Autodesk Inventor part; units mm, degrees
ref_plane "YZ Plane" through (0, 0, 0) normal (1, 0, 0) x (0, 1, 0)
ref_plane "XZ Plane" through (0, 0, 0) normal (0, 1, 0) x (-1, 0, 0)
ref_plane "XY Plane" through (0, 0, 0) normal (0, 0, 1) x (1, 0, 0)
sketch "Sketch1" plane through (0, 0, 0) normal (0, 0, 1) x (1, 0, 0)
  line L0 (-5, 12.5) -> (5, 12.5)
  line L1 (5, 12.5) -> (5, 2.5)
  line L2 (5, 2.5) -> (-5, 2.5)
  line L3 (-5, 2.5) -> (-5, 12.5)
  line L4 (-6.5, 1) -> (-6.5, 14)
  line L5 (6.5, 1) -> (-6.5, 1)
  line L6 (6.5, 14) -> (6.5, 1)
  line L7 (-6.5, 14) -> (6.5, 14)
  line L8 (-5, 2.5) -> (5, 2.5)
  line L9 (5, 2.5) -> (5, 12.5)
  line L10 (5, 12.5) -> (-5, 12.5)
  line L11 (-5, 12.5) -> (-5, 2.5)
  line L12 (4.1303, 3.3697) -> (-4.1303, 3.3697)
  line L13 (-4.1303, 3.3697) -> (-4.1303, 11.6303)
  line L14 (-4.1303, 11.6303) -> (4.1303, 11.6303)
  line L15 (4.1303, 11.6303) -> (4.1303, 3.3697)
  line L16 (-4.1303, 3.3697) -> (4.1303, 11.6303) construction
  point P0 (0, 0)
  point P1 (0, 7.5)
extrude "Extrusion1" add sketch "Sketch1" along normal blind 30 contours L0 L1 L2 L3
sketch "Sketch2" plane through (0, 0, 30) normal (0, 0, 1) x (1, 0, 0)
  line L0 (-5, 2.5) -> (5, 2.5)
  line L1 (5, 2.5) -> (5, 12.5)
  line L2 (5, 12.5) -> (-5, 12.5)
  line L3 (-5, 12.5) -> (-5, 2.5)
  line L4 (3.175, 4.325) -> (-3.175, 4.325)
  line L5 (-3.175, 4.325) -> (-3.175, 10.675)
  line L6 (-3.175, 10.675) -> (3.175, 10.675)
  line L7 (3.175, 10.675) -> (3.175, 4.325)
  line L8 (-3.175, 4.325) -> (3.175, 10.675) construction
  point P0 (0, 0)
  point P1 (0, 7.5)
extrude "Extrusion2" add sketch "Sketch2" along normal blind 1
properties part number "arm-seg1"
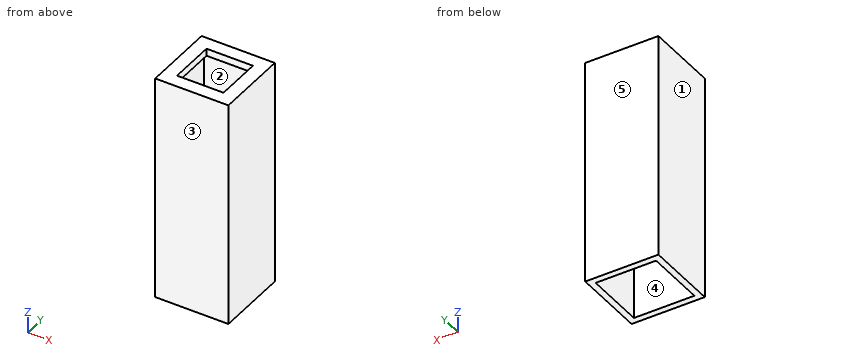
Geometry: final body of the model. Coordinates: model frame, mm. Face numbers are marked on the shaded views. A direction names the side the tool comes from. Give positions to 0.01 mm unless a question says otherwise; leave off trailing zeros. Write each loop counter-clockwise with the first axis right and the second up, starting at its lowest first coordinate (ties: lowest second). Pieces come first, ordered by that corner, then holes. Notation, with made-up numbers: (71.25, 55.25) - (79.25, 55.25) arc R18 cw to (79.25, 80.25) - close; hole circle Ø2 at (41, -39). An arc over 180 degrees is marked (long way). Return JSON: item names as keys, results as strings. Group by question number.
1) Set-up query: the marked faces 1 and 2. Return all of +Z, -Z, +X, -X, +Y, -Y with unobstructed straight access to the full face (end or side cutting, diameter ignored); none if empty.
2) Mould query, pull axis Y, two halves, no side actions, for the marked faces 3, 4 and 5. Classes: released by +Y, released by -Y, zero draft, split by the parting line, or undercut.
3) Line query: line 1 (Y direction, x = -2.5, z = 3.5); line 2 (X direction, y = 4, z = 20); line 3 (Z direction, x = 3.5, y = 10.75). Output: solid intervals per line, ascending.
4) Section B-B on y = 8.5. Return the cut outline in (x, z) (3 decimals), plus the area to 3 significant figures.
5) Section C-C on x = -0.75. Return the cut outline in (y, z) (3 decimals).
6) Section D-D on x = 3.75. Return the cut outline in (y, z).
7) Section A-A on z = 24.5. Return the cut outline in (x, y).
8) First-contact query: P1, Ø2.5, axis at x = -1, y = 8.5, coming from the -Z side. Flat tip, straight axial feed; report the tip coordinate or a pass-through.
Filled in:
{
 "1": {"face 1": "+Z, -Z, -X, +Y, -Y", "face 2": "-Z"},
 "2": {"face 3": "released by -Y", "face 4": "undercut", "face 5": "released by +Y"},
 "3": {"line 1": "y = 2.5 to 3.37, 11.63 to 12.5", "line 2": "x = -5 to -4.13, 4.13 to 5", "line 3": "z = 30 to 31"},
 "4": {"outline": "(-5, 0) - (-4.13, 0) - (-4.13, 30) - (-3.175, 30) - (-3.175, 31) - (-5, 31) - close; (3.175, 30) - (4.13, 30) - (4.13, 0) - (5, 0) - (5, 31) - (3.175, 31) - close", "area": "55.8 mm^2"},
 "5": {"outline": "(2.5, 0) - (3.37, 0) - (3.37, 30) - (4.325, 30) - (4.325, 31) - (2.5, 31) - close; (10.675, 30) - (11.63, 30) - (11.63, 0) - (12.5, 0) - (12.5, 31) - (10.675, 31) - close"},
 "6": {"outline": "(2.5, 0) - (3.37, 0) - (3.37, 30) - (11.63, 30) - (11.63, 0) - (12.5, 0) - (12.5, 31) - (2.5, 31) - close"},
 "7": {"outline": "(-5, 2.5) - (5, 2.5) - (5, 12.5) - (-5, 12.5) - close; hole (-4.13, 3.37) - (4.13, 3.37) - (4.13, 11.63) - (-4.13, 11.63) - close"},
 "8": {"P1": "passes through"}
}
